from build123d import *

# Parameters (mm, degrees)
F0_W     = 10
F0_H     = 10
F0_W_2   = 9.2
F0_H_2   = 9.2
F1_DEPTH = 70
F2_R     = 1.5
F3_DEPTH = 25


with BuildPart() as f1:
    # F0 (on Top) → F1 (new body)
    with BuildSketch(Plane.XY):
        Rectangle(F0_W, F0_H)
        Rectangle(F0_W_2, F0_H_2, mode=Mode.SUBTRACT)
    extrude(amount=F1_DEPTH)

    # F2 (on face) → F3 (cut)
    with BuildSketch(Plane(origin=(0, 5, 0), x_dir=(-1, 0, 0), z_dir=(0, 1, 0))):
        with Locations((0, 60)):
            Circle(F2_R)
        with Locations((0, 50)):
            Circle(F2_R)
        with Locations((0, 40)):
            Circle(F2_R)
        with Locations((0, 30)):
            Circle(F2_R)
        with Locations((0, 20)):
            Circle(F2_R)
        with Locations((0, 10)):
            Circle(F2_R)
    extrude(amount=-F3_DEPTH, mode=Mode.SUBTRACT)


solid = f1.part
The model under review builds one solid part; all positions refer to its coordinate system, in mm. A direction names the side the tool comes from. Round coordinates to 2 decimals unless told otherwise and drop trailing zeros. Write each loop counter-clockwise with the first axis right and the second up, starting at its lowest first coordinate (ties: lowest second). Pieces come first, ordered by that corner, then holes. Notation, with made-up numbers: M 44.5,71.25 L 92.5,71.25 A15 cw 92.5,89.25 Z; hole C 13.5,-29.75 d11. An arc over 180 degrees is marked long. Answer as CSV lines item,"result". Start each with the question number.
Q1. Clearance check with a flat-ended pin moving along its axis: P1, Ø3.5, axis at x = 0, z = 30, coming from the +Y side. State where the tip first meets the part, or that it passes through.
Q2. Consider section A-A, the plane z = 53. Give the boundary of the cut face in (x, y).
Q3. Consider section B-B, the plane x = -2.25. Give the boundary of the cut face in (y, z), then the cut area to 3 significant figures.
Q4. The part is to be moulded in two halves that separate along Y. For faces 1 (the face through (0.325, 4.803, 8.536)), 2 (the face through (0, -5, 35)), 3 (the face through (-4.6, 0, 35)), say which applies: +Y half, -Y half, draft (parallel to the pull), parting line (faces both ways), or undercut.
Q5. Tool access review of faces 4 (the face through (0.325, -4.797, 8.536)), 5 (the face through (0, -4.6, 35)): name each direction out of +Z, -Z, +X, -X, +Y, -Y from which nothing blocks a thin tool from reaching the whole face with its end or side.
Q6. Consider section D-D, the plane z = 30. Give the boundary of the cut face in (x, y).
Q7. Wall thickness on line 1 along Y through (x, z) = (-3.5, 48): over which ranges is the line inside the solid? List them lowest first.
Result set:
1,P1,"stops at y = 5"
2,outline,"M -5,-5 L 5,-5 L 5,5 L -5,5 Z; hole M -4.6,-4.6 L 4.6,-4.6 L 4.6,4.6 L -4.6,4.6 Z"
3,outline,"M -5,0 L -4.6,0 L -4.6,70 L -5,70 Z; M 4.6,0 L 5,0 L 5,70 L 4.6,70 Z"
3,area,"56.0 mm²"
4,face 1,"draft"
4,face 2,"-Y half"
4,face 3,"undercut"
5,face 4,"+Y, -Y"
5,face 5,"+Z, -Z"
6,outline,"M -5,-5 L -1.5,-5 L -1.5,-4.6 L -4.6,-4.6 L -4.6,4.6 L -1.5,4.6 L -1.5,5 L -5,5 Z; M 1.5,-5 L 5,-5 L 5,5 L 1.5,5 L 1.5,4.6 L 4.6,4.6 L 4.6,-4.6 L 1.5,-4.6 Z"
7,line 1,"y = -5 to -4.6, 4.6 to 5"
